Input: dimensioned drawing with shaded views. Units: mm. Origin: part minimum x, y, z. A direction names the side the tool comes from. Give positions to 0.01 mm unless a question says otherwise; leave off trailing zeros. Order: outer loops, then holes, each group sorted by start corner. A loop starts at its lowest first (then second) coordinate and runs counter-clockwise, first axis right, second up.
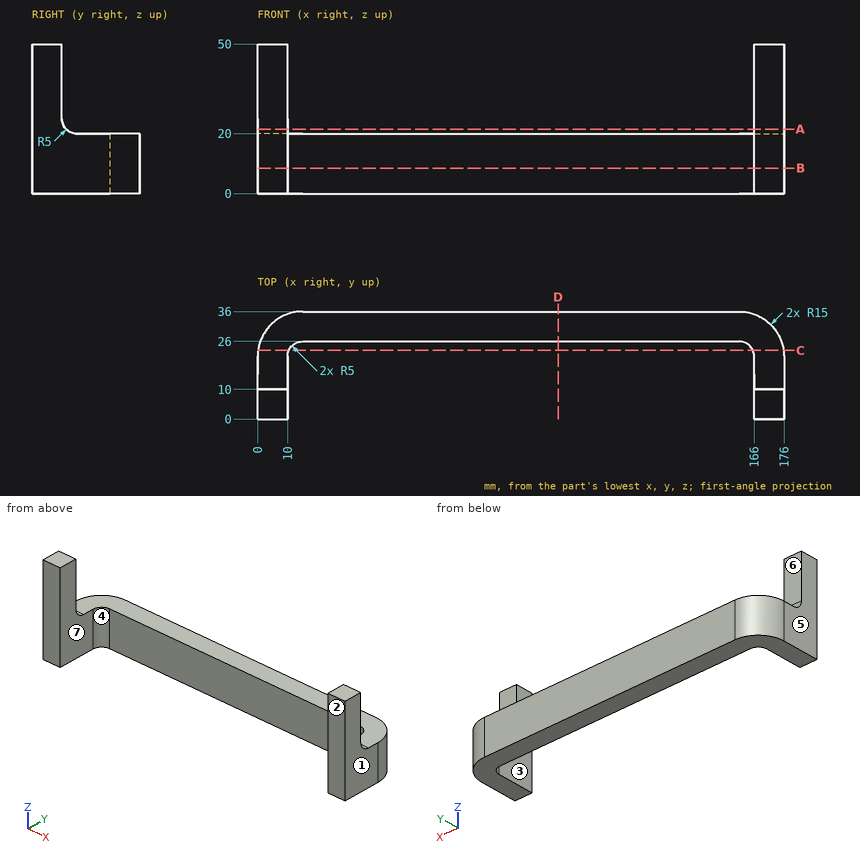
1) Draft query along X for the marked faces 1, 2, 3 and 4. Return one class per face: +X half, -X half, draft (parallel to the pull), parting line (faces both ways), or undercut.
Report:
face 1: +X half
face 2: draft
face 3: undercut
face 4: undercut
2) Section query A-A, the plane z = 21.5. Return the cut outline in (x, y).
Report:
outline: (0, 0) - (10, 0) - (10, 11.43) - (0, 11.43) - close; (166, 0) - (176, 0) - (176, 11.43) - (166, 11.43) - close
3) Section query B-B, the plane z = 8.5. Return the cut outline in (x, y).
Report:
outline: (0, 0) - (10, 0) - (10, 21) arc R5 cw to (15, 26) - (161, 26) arc R5 cw to (166, 21) - (166, 0) - (176, 0) - (176, 21) arc R15 ccw to (161, 36) - (15, 36) arc R15 ccw to (0, 21) - close
4) Section query D-D, the plane x = 100.5. Return the cut outline in (y, z).
Report:
outline: (26, 0) - (36, 0) - (36, 20) - (26, 20) - close
5) Pin query (flat end, axial travel): pin 1 (2 mm diameter, centred on y = 27, z = 5.5, fed in from +X); pin 2 (22 mm diameter, centred on x = 61.5, z = 12.5, fed in from -Y); pin 3 (3 mm diameter, centred on x = 170, z = 34.5, fed in from +Y). Return the tip coordinate at first contact, or that it passes through.
Report:
pin 1: stops at x = 175.14
pin 2: stops at y = 26
pin 3: stops at y = 10
6) Material intervals for L1, parallel to X at y = 5, z = 30; L2, parallel to Z at x = 118, y = 30; L3, parallel to Y at x = 58, z = 8.5, sorted ascending.
Report:
L1: x = 0 to 10, 166 to 176
L2: z = 0 to 20
L3: y = 26 to 36
7) Section query C-C, the plane y = 23. Return the cut outline in (x, z).
Report:
outline: (0.13, 0) - (10.42, 0) - (10.42, 20) - (0.13, 20) - close; (165.58, 0) - (175.87, 0) - (175.87, 20) - (165.58, 20) - close
8) Reachability of the marked faces 5, 6 and 7 from +Z, -Z, +X, -X, +Y, -Y: full face, straight path, thin tool, end or side. Return the list, or none.
Report:
face 5: +Z, -Z, -X, +Y, -Y
face 6: +Z, +X, -X, +Y
face 7: +Z, -Z, -Y
